Here's how the part is built. I have some questions about the finished solid (model axes, mm). A direction names the side the tool comes from. Round coordinates to 2 decimals unless told otherwise and drop trailing zeros. Write each loop counter-clockwise with the first axis right and the second up, starting at its lowest first coordinate (ties: lowest second). Pieces come first, ordered by that corner, then holes. Notation, with made-up numbers: (-0.5, 51.25) - (16.5, 51.25) arc R17 ccw to (16.5, 55.25) - close; hole circle Ø10 at (73, -1.75). An arc over 180 degrees is marked (long way). One line per item, written item: value. Start each with the question number.
Item 1: If I drill on line 1 (X direction, y = 1.1, z = 0); line 2 (X direction, y = -5, z = 0); line 3 (Y direction, x = 18.5, z = -9), over which ranges is the centre line in solid material (lowest first)?
Item 2: For faces 4 (the face through (-21, -11, -28)), 5 (the face through (-43.788, 1.972, -44.417)), which set-ups out of +Z, -Z, +X, -X, +Y, -Y let a thin tool reach every point of the face, with its end or its side?
Item 3: Imagine slicing it at A-A, the plane x = 0. Please give me the cut outline in (y, z), then the cut area to 3 significant figures.
Item 4: Imagine slicing it at C-C, the plane z = 59. Please give me the cut outline in (x, y), then the cut area to 3 significant figures.
Item 5: For P1, Ø8, axis at x = 41.72, z = 41.72, coming from the -Y side; P2, Ø12, axis at x = 36, y = -17.5, coming from the +Z side; P3, Ø4, axis at x = -59, z = 0, coming from the +Y side; P4, Ø1.5, axis at y = -1.5, z = -18, coming from the +X side, each with a flat end and sliding along its axis, tell me the tip position at first contact or that it passes through.
Item 6: Thinking about a two-plate mould opening in Z: for faces 1 (the face through (-62.32, 1.97, -0.74)), 2 (the face through (-42.594, 1.972, -55.55)), 3 (the face through (1, 4, -1)), which applies, released by +Z, released by -Z, zero draft, split by the parting line, or undercut?
Item 7: Imagine slicing it at B-B, the plane x = -59. Please give me the cut outline in (y, z).
Item 8: Imagine slicing it at D-D, the plane y = -3.75. Please give me the cut outline in (x, z), then the cut area to 3 significant figures.
```python
from build123d import *

# Parameters (mm, degrees)
SKETCH_1_R      = 70
SKETCH_1_R_2    = 3.4
EXTRUDE_1_DEPTH = 4
SKETCH_2_R      = 40
SKETCH_2_R_2    = 35
EXTRUDE_2_DEPTH = 21
FILLET_2_R      = 1


with BuildPart() as part:
    # Эскиз1 → Бобышка-Вытянуть1 (new body)
    with BuildSketch(Plane(origin=(0, 0, 0), x_dir=(1, 0, 0), z_dir=(0, 1, 0))):
        with Locations(Location((0, 0, 0), (0, 0, 270))):
            Circle(SKETCH_1_R)
        with Locations(Location((59, 0, 0), (0, 0, 270))):
            Circle(SKETCH_1_R_2, mode=Mode.SUBTRACT)
        with Locations(Location((41.71930009, -41.71930009, 0), (0, 0, 270))):
            Circle(SKETCH_1_R_2, mode=Mode.SUBTRACT)
        with Locations(Location((0, -59, 0), (0, 0, 270))):
            Circle(SKETCH_1_R_2, mode=Mode.SUBTRACT)
        with Locations(Location((-41.71930009, -41.71930009, 0), (0, 0, 270))):
            Circle(SKETCH_1_R_2, mode=Mode.SUBTRACT)
        with Locations(Location((-59, 0, 0), (0, 0, 270))):
            Circle(SKETCH_1_R_2, mode=Mode.SUBTRACT)
        with Locations(Location((-41.71930009, 41.71930009, 0), (0, 0, 270))):
            Circle(SKETCH_1_R_2, mode=Mode.SUBTRACT)
        with Locations(Location((0, 59, 0), (0, 0, 270))):
            Circle(SKETCH_1_R_2, mode=Mode.SUBTRACT)
        with Locations(Location((41.71930009, 41.71930009, 0), (0, 0, 270))):
            Circle(SKETCH_1_R_2, mode=Mode.SUBTRACT)
    extrude(amount=EXTRUDE_1_DEPTH)

    # Эскиз2 → Бобышка-Вытянуть2 (add)
    with BuildSketch(Plane(origin=(0, 0, 0), x_dir=(1, 0, 0), z_dir=(0, 1, 0))):
        with Locations(Location((0, 0, 0), (0, 0, 270))):
            Circle(SKETCH_2_R)
        with Locations(Location((0, 0, 0), (0, 0, 270))):
            Circle(SKETCH_2_R_2, mode=Mode.SUBTRACT)
    extrude(amount=-EXTRUDE_2_DEPTH)

    # Скругление2
    fillet_2_edges = [part.edges().sort_by_distance(p)[0] for p in [
        (0, 0, -35),
        (0, 0, -40),
    ]]
    fillet(fillet_2_edges, radius=FILLET_2_R)


solid = part.part
```
Values follow:
1. line 1: x = -70 to -62.4, -55.6 to 55.6, 62.4 to 70
1. line 2: x = -40 to -35, 35 to 40
1. line 3: y = 0 to 4
2. face 4: -Y
2. face 5: +Y, -Y
3. outline: (-21, -40) - (-1, -40) arc R1 cw to (0, -41) - (0, -55.6) - (4, -55.6) - (4, 55.6) - (0, 55.6) - (0, 41) arc R1 cw to (-1, 40) - (-21, 40) - (-21, 35) - (-1, 35) arc R1 cw to (0, 34) - (0, -34) arc R1 cw to (-1, -35) - (-21, -35) - close; (0, -70) - (4, -70) - (4, -62.4) - (0, -62.4) - close; (0, 62.4) - (4, 62.4) - (4, 70) - (0, 70) - close
3. area: 716 mm^2
4. outline: (-37.67, 0) - (-3.4, 0) - (-3.4, 4) - (-37.67, 4) - close; (3.4, 0) - (37.67, 0) - (37.67, 4) - (3.4, 4) - close
4. area: 274 mm^2
5. P1: stops at y = 0
5. P2: stops at z = 26.46
5. P3: passes through
5. P4: stops at x = 36.09
6. face 1: undercut
6. face 2: split by the parting line
6. face 3: zero draft
7. outline: (0, -37.67) - (4, -37.67) - (4, -3.4) - (0, -3.4) - close; (0, 3.4) - (4, 3.4) - (4, 37.67) - (0, 37.67) - close
8. outline: circle Ø80 at (0, 0); hole circle Ø70 at (0, 0)
8. area: 1,180 mm^2
